Can you work these out from the model? Positions are in its coordinate system, mm. Face numbers are marked on the shaded views. A direction names the side the tool comes from. Give positions to 0.01 mm unless a question says otherwise; leave off trailing zeros. Write each loop counter-clockwise with the first axis right and the second up, starting at its lowest first coordinate (ties: lowest second). Pieces come first, ordered by that corner, then holes. Notation, with made-up numbers: M 80,89 L 99,89 A15 cw 99,107 Z; hole C -9.75,83.5 d5. An arc over 180 degrees is marked long. Use CSV: the item, a comma, the result in double quotes. Start each with the question number.
from build123d import *

# Parameters (mm, degrees)
BOSS_EXTRUDE1_DEPTH = 5
SKETCH2_R           = 19
BOSS_EXTRUDE2_DEPTH = 5
CUT_EXTRUDE1_DEPTH  = 3.5
SKETCH4_R           = 6
CUT_EXTRUDE2_DEPTH  = 11


with BuildPart() as part:
    # Sketch1 → Boss-Extrude1 (new body)
    with BuildSketch(Plane.XY):
        Polygon((8.766334056, 10.506254671), (-4.715516416, 12.844995326), (-13.481850472, 2.338740655), (-8.766334056, -10.506254671), (4.715516416, -12.844995326), (13.481850472, -2.338740655), align=None)
    extrude(amount=BOSS_EXTRUDE1_DEPTH)

    # Sketch2 → Boss-Extrude2 (add)
    with BuildSketch(Plane.XY.offset(5)):
        Circle(SKETCH2_R)
    extrude(amount=BOSS_EXTRUDE2_DEPTH)

    # Sketch3 → Cut-Extrude1 (cut)
    with BuildSketch(Plane.XY.offset(10)):
        with BuildLine():
            Line((7.666666546, -3.670452843), (14.211444215, -3.120072648))
            ThreePointArc((14.211444215, -3.120072648), (16.499429689, -0.741033748), (14.433922262, 1.833530816))
            Line((14.433922262, 1.833530816), (7.964835621, 2.968399152))
            ThreePointArc((7.964835621, 2.968399152), (7.544489735, 3.915440541), (7.012038678, 4.80430157))
            Line((7.012038678, 4.80430157), (9.807784283, 10.74743539))
            ThreePointArc((9.807784283, 10.74743539), (8.89146974, 13.918407845), (5.629078153, 13.4169103))
            Line((5.629078153, 13.4169103), (1.411708737, 8.381949561))
            ThreePointArc((1.411708737, 8.381949561), (0.381373892, 8.49144004), (-0.654627868, 8.474754413))
            Line((-0.654627868, 8.474754413), (-4.403659932, 13.867508039))
            ThreePointArc((-4.403659932, 13.867508039), (-7.607959927, 14.659442582), (-8.804846066, 11.583379783))
            Line((-8.804846066, 11.583379783), (-6.553126885, 5.413550409))
            ThreePointArc((-6.553126885, 5.413550409), (-7.163115843, 4.575999499), (-7.666666546, 3.670452843))
            Line((-7.666666546, 3.670452843), (-14.211444215, 3.120072648))
            ThreePointArc((-14.211444215, 3.120072648), (-16.499429618, 0.741035318), (-14.433925359, -1.833530273))
            Line((-14.433925359, -1.833530273), (-7.964835621, -2.968399152))
            ThreePointArc((-7.964835621, -2.968399152), (-7.544489735, -3.915440541), (-7.012038678, -4.80430157))
            Line((-7.012038678, -4.80430157), (-9.807784283, -10.74743539))
            ThreePointArc((-9.807784283, -10.74743539), (-8.891470467, -13.918407381), (-5.629079261, -13.416911623))
            Line((-5.629079261, -13.416911623), (-1.411708737, -8.381949561))
            ThreePointArc((-1.411708737, -8.381949561), (-0.381373892, -8.49144004), (0.654627868, -8.474754413))
            Line((0.654627868, -8.474754413), (4.403659932, -13.867508039))
            ThreePointArc((4.403659932, -13.867508039), (7.607959014, -14.659443056), (8.804846772, -11.583381715))
            Line((8.804846772, -11.583381715), (6.553126885, -5.413550409))
            ThreePointArc((6.553126885, -5.413550409), (7.163115843, -4.575999499), (7.666666546, -3.670452843))
        make_face()
    extrude(amount=-CUT_EXTRUDE1_DEPTH, mode=Mode.SUBTRACT)

    # Sketch4 → Cut-Extrude2 (cut, through all)
    with BuildSketch(Plane(origin=(0, 0, 0), x_dir=(-1, 0, 0), z_dir=(0, 0, -1))):
        Circle(SKETCH4_R)
    extrude(amount=-CUT_EXTRUDE2_DEPTH, mode=Mode.SUBTRACT)


solid = part.part
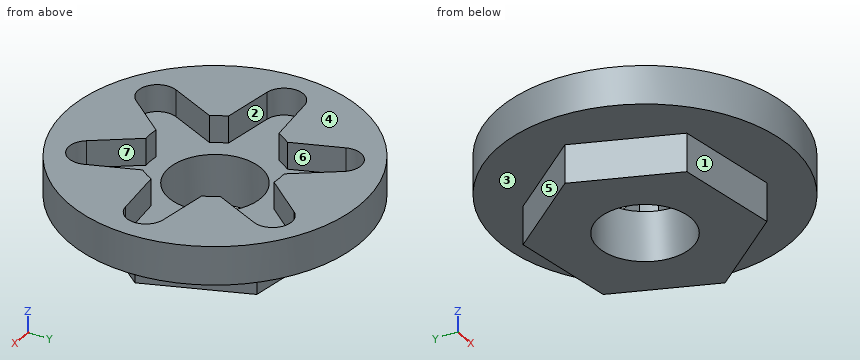
(1) I want a section at B-B (z = 2). Write out the boundary of the cut face in (x, y) (3 decimals).
(2) I want a section at D-D (x = 12). Write out the boundary of the cut face in (y, z).
(3) Thinking about a two-plate mould opening in X: for the marked faces 4, 5, 6 and 7, which applies, released by +X, released by -X, zero draft, split by the parting line, or undercut?
(4) Which directions (+Z, -Z, +X, -X, +Y, -Y) give clear straight access to the entire face, cutting with the end or side of a thin tool? Please do the marked faces 1, 2 and 3.
(5) I want a section at C-C (y = -9). Write out the boundary of the cut face in (x, z).
(6) Please list where these lines run through material, in increasing order: L1, parallel to Y at x = 9, z = 8.5 (3 decimals); L2, parallel to X at y = 12, z = 9.25; L3, parallel to Z at x = 12, y = -5.5. Write a range as [from, to].
(7) Will these pins go through, and if not, where does the flat tip stop? pin 1 Ø3 at (x, z) = (8, 2.5) entering from +Y; pin 2 Ø1.5 at (x, z) = (9, 4.5) entering from -Y; pin 3 Ø9.5 at (x, y) = (0, 0) entering from -Z; pin 4 Ø3 at (x, y) = (6.5, -13.5) entering from -Z.
(8) I want a section at A-A (x = 0). Write out the boundary of the cut face in (y, z).
Geometry results:
1,outline,"M -13.482,2.339 L -8.766,-10.506 L 4.716,-12.845 L 13.482,-2.339 L 8.766,10.506 L -4.716,12.845 Z; hole C 0,0 d12"
2,outline,"M -14.73,5 L -4.11,5 L -4.11,0 L 1.7,0 L 1.7,5 L 14.73,5 L 14.73,10 L 2.26,10 L 2.26,6.5 L -3.31,6.5 L -3.31,10 L -14.73,10 Z"
3,face 4,"zero draft"
3,face 5,"released by -X"
3,face 6,"undercut"
3,face 7,"undercut"
4,face 1,"-Z, -X, -Y"
4,face 2,"+Z"
4,face 3,"-Z"
5,outline,"M -16.73,5 L -9.32,5 L -9.32,0 L 7.92,0 L 7.92,5 L 16.73,5 L 16.73,10 L 7.86,10 L 7.86,6.5 L 1.02,6.5 L 1.02,10 L -1.93,10 L -1.93,6.5 L -8.99,6.5 L -8.99,10 L -16.73,10 Z"
6,L1,"y = [-16.733, -3.558], [2.787, 9.03], [13.845, 16.733]"
6,L2,"x = [-14.73, -8.92], [-3.11, 4.44], [10.04, 14.73]"
6,L3,"z = [5, 10]"
7,pin 1,"stops at y = 10.9"
7,pin 2,"stops at y = -17.02"
7,pin 3,"passes through"
7,pin 4,"stops at z = 5"
8,outline,"M -19,5 L -12.03,5 L -12.03,0 L -6,0 L -6,6.5 L -8.5,6.5 L -8.5,10 L -19,10 Z; M 6,0 L 12.03,0 L 12.03,5 L 19,5 L 19,10 L 8.5,10 L 8.5,6.5 L 6,6.5 Z"
